Geometry: final body of the model. Coordinates: model frame, mm. A direction names the side the tool comes from. Give positions to 0.01 mm unless a question says otherwise; leave off trailing zeros. Loops run counter-clockwise (first coordinate to the right, second up) from the corner with the lowest first, then second, coordinate; pieces in that order, holes last.
```python
from build123d import *

# Parameters (mm, degrees)
BOSS_EXTRUDE1_DEPTH          = 29.21
SHELL1_T                     = -2.54
FILLET1_R                    = 6.35
BOSS_EXTRUDE2_DEPTH          = 38.1
SKETCH3_R                    = 2.8067
CUT_EXTRUDE1_DEPTH           = 4.7
CUT_EXTRUDE1_DRAFT           = -8
CUT_EXTRUDE1_PROFILE_2_DEPTH = 4.7
CUT_EXTRUDE1_PROFILE_2_DRAFT = -8
CUT_EXTRUDE1_PROFILE_3_DEPTH = 4.7
CUT_EXTRUDE1_PROFILE_3_DRAFT = -8
CUT_EXTRUDE1_PROFILE_4_DEPTH = 4.7
CUT_EXTRUDE1_PROFILE_4_DRAFT = -8
SKETCH5_W                    = 45.253999916
SKETCH5_H                    = 45.253999916
CUT_EXTRUDE5_DEPTH           = 38.1


with BuildPart() as part:
    # Sketch1 → Boss-Extrude1 (new, symmetric)
    with BuildSketch(Plane.XY):
        Polygon((-32.258, -32.258), (-32.258, -11.938), (-32.258, 11.938), (-32.258, 32.258), (32.258, 32.258), (32.258, -32.258), align=None)
    extrude(amount=BOSS_EXTRUDE1_DEPTH, both=True)

    # Shell1
    shell1_openings = [part.faces().sort_by_distance(p)[0] for p in [
        (0, 0, 29.21),
    ]]
    offset(amount=SHELL1_T, openings=shell1_openings, kind=Kind.INTERSECTION)

    # Fillet1
    fillet1_edges = [part.edges().sort_by_distance(p)[0] for p in [
        (-32.258, -32.258, 0),
        (-32.258, 32.258, 0),
        (32.258, 32.258, 0),
        (32.258, -32.258, 0),
        (-29.718, -29.718, 1.27),
        (29.718, -29.718, 1.27),
        (29.718, 29.718, 1.27),
        (-29.718, 29.718, 1.27),
        (-32.258, 0, -29.21),
        (0, 32.258, -29.21),
        (32.258, 0, -29.21),
        (0, -32.258, -29.21),
    ]]
    fillet(fillet1_edges, radius=FILLET1_R)

    # Sketch2 → Boss-Extrude2 (add)
    with BuildSketch(Plane.XY.offset(-26.67)):
        with BuildLine():
            Line((-20.828, -20.828), (-29.718, -20.828))
            Line((-29.718, -20.828), (-29.718, -23.368))
            ThreePointArc((-29.718, -23.368), (-27.858128061, -27.858128061), (-23.368, -29.718))
            Line((-23.368, -29.718), (-20.828, -29.718))
            Line((-20.828, -29.718), (-20.828, -20.828))
        make_face()
        with BuildLine():
            ThreePointArc((-29.718, 23.368), (-27.858128061, 27.858128061), (-23.368, 29.718))
            Line((-23.368, 29.718), (-20.828, 29.718))
            Line((-20.828, 29.718), (-20.828, 20.828))
            Line((-20.828, 20.828), (-29.718, 20.828))
            Line((-29.718, 20.828), (-29.718, 23.368))
        make_face()
        with BuildLine():
            ThreePointArc((29.718, 23.368), (27.858128061, 27.858128061), (23.368, 29.718))
            Line((23.368, 29.718), (20.828, 29.718))
            Line((20.828, 29.718), (20.828, 20.828))
            Line((20.828, 20.828), (29.718, 20.828))
            Line((29.718, 20.828), (29.718, 23.368))
        make_face()
        with BuildLine():
            ThreePointArc((23.368, -29.718), (27.858128061, -27.858128061), (29.718, -23.368))
            Line((29.718, -23.368), (29.718, -20.828))
            Line((29.718, -20.828), (20.828, -20.828))
            Line((20.828, -20.828), (20.828, -29.718))
            Line((20.828, -29.718), (23.368, -29.718))
        make_face()
    extrude(amount=BOSS_EXTRUDE2_DEPTH)


with BuildPart() as cut_extrude1_tool:
    # Sketch3 → Cut-Extrude1 (with draft: the straight prism first)
    with BuildSketch(Plane.XY.offset(11.43)):
        with Locations((-25.4, -25.4)):
            Circle(SKETCH3_R)
    extrude(amount=-CUT_EXTRUDE1_DEPTH)
    # Cut-Extrude1: the draft: its side faces are tilted about the plane it starts from
    cut_extrude1_sides = [cut_extrude1_tool.faces().sort_by_distance(p)[0] for p in [
        (-28.2067, -25.4, 9.08),
    ]]
    draft(cut_extrude1_sides, Plane.XY.offset(11.43), CUT_EXTRUDE1_DRAFT)


with BuildPart() as part_1:
    add(part.part)

    # Cut-Extrude1: cut by cut_extrude1_tool
    add(cut_extrude1_tool.part, mode=Mode.SUBTRACT)


with BuildPart() as cut_extrude1_profile_2_tool:
    # Sketch3 → Cut-Extrude1 profile 2 (with draft: the straight prism first)
    with BuildSketch(Plane.XY.offset(11.43)):
        with Locations((-25.4, 25.4)):
            Circle(SKETCH3_R)
    extrude(amount=-CUT_EXTRUDE1_PROFILE_2_DEPTH)
    # Cut-Extrude1 profile 2: the draft: its side faces are tilted about the plane it starts from
    cut_extrude1_profile_2_sides = [cut_extrude1_profile_2_tool.faces().sort_by_distance(p)[0] for p in [
        (-28.2067, 25.4, 9.08),
    ]]
    draft(cut_extrude1_profile_2_sides, Plane.XY.offset(11.43), CUT_EXTRUDE1_PROFILE_2_DRAFT)


with BuildPart() as part_2:
    add(part_1.part)

    # Cut-Extrude1 profile 2: cut by cut_extrude1_profile_2_tool
    add(cut_extrude1_profile_2_tool.part, mode=Mode.SUBTRACT)


with BuildPart() as cut_extrude1_profile_3_tool:
    # Sketch3 → Cut-Extrude1 profile 3 (with draft: the straight prism first)
    with BuildSketch(Plane.XY.offset(11.43)):
        with Locations((25.4, 25.4)):
            Circle(SKETCH3_R)
    extrude(amount=-CUT_EXTRUDE1_PROFILE_3_DEPTH)
    # Cut-Extrude1 profile 3: the draft: its side faces are tilted about the plane it starts from
    cut_extrude1_profile_3_sides = [cut_extrude1_profile_3_tool.faces().sort_by_distance(p)[0] for p in [
        (22.5933, 25.4, 9.08),
    ]]
    draft(cut_extrude1_profile_3_sides, Plane.XY.offset(11.43), CUT_EXTRUDE1_PROFILE_3_DRAFT)


with BuildPart() as part_3:
    add(part_2.part)

    # Cut-Extrude1 profile 3: cut by cut_extrude1_profile_3_tool
    add(cut_extrude1_profile_3_tool.part, mode=Mode.SUBTRACT)


with BuildPart() as cut_extrude1_profile_4_tool:
    # Sketch3 → Cut-Extrude1 profile 4 (with draft: the straight prism first)
    with BuildSketch(Plane.XY.offset(11.43)):
        with Locations((25.4, -25.4)):
            Circle(SKETCH3_R)
    extrude(amount=-CUT_EXTRUDE1_PROFILE_4_DEPTH)
    # Cut-Extrude1 profile 4: the draft: its side faces are tilted about the plane it starts from
    cut_extrude1_profile_4_sides = [cut_extrude1_profile_4_tool.faces().sort_by_distance(p)[0] for p in [
        (22.5933, -25.4, 9.08),
    ]]
    draft(cut_extrude1_profile_4_sides, Plane.XY.offset(11.43), CUT_EXTRUDE1_PROFILE_4_DRAFT)


with BuildPart() as part_4:
    add(part_3.part)

    # Cut-Extrude1 profile 4: cut by cut_extrude1_profile_4_tool
    add(cut_extrude1_profile_4_tool.part, mode=Mode.SUBTRACT)

    # Sketch5 → Cut-Extrude5 (cut)
    with BuildSketch(Plane.XY.offset(11.43)):
        Rectangle(SKETCH5_W, SKETCH5_H)
    extrude(amount=-CUT_EXTRUDE5_DEPTH, mode=Mode.SUBTRACT)


solid = part_4.part
```
Q1. Section query A-A, the plane x = -7.5. Return loops of the section in (y, z).
Q2. Mould query, pull axis Y, two halves, no side actions, for faces 1 (the face through (30.45, -0.36, -27.3)), 2 (the face through (-30.447, -30.348, 3.539)), 3 (the face through (-22.627, -22, -7)). Classes: +Y half, -Y half, draft (parallel to the pull), parting line (faces both ways), or undercut.
Q3. Section query B-B, the plane z = 1. Return loops of the section in (x, y).
Q4. Reachability of faces 4 (the face through (20.828, 26, -8)), 5 (the face through (3, -31, 29.21)) from +Z, -Z, +X, -X, +Y, -Y: full face, straight path, thin tool, end or side. Return the list, or none.
Q5. Pin query (flat end, axial travel): pin 1 Ø10 at (x, y) = (24, 8.5) entering from +Z; pin 2 Ø7 at (x, y) = (25, -27.5) entering from +Z; pin 3 Ø4.5 at (x, y) = (27, 23.5) entering from +Z. Return the tip coordinate at first contact, or that it passes through.
Q6. Material intervals for probe 1 along X at (y, z) = (11.5, -16); probe 2 along Y at (x, z) = (-25, 2), sorted ascending.
Resolved:
1. outline: (-32.26, -22.86) arc R6.35 ccw to (-25.91, -29.21) - (25.91, -29.21) arc R6.35 ccw to (32.26, -22.86) - (32.26, 29.21) - (29.72, 29.21) - (29.72, -26.67) - (-29.72, -26.67) - (-29.72, 29.21) - (-32.26, 29.21) - close
2. face 1: draft
2. face 2: -Y half
2. face 3: undercut
3. outline: (-32.26, -25.91) arc R6.35 ccw to (-25.91, -32.26) - (25.91, -32.26) arc R6.35 ccw to (32.26, -25.91) - (32.26, 25.91) arc R6.35 ccw to (25.91, 32.26) - (-25.91, 32.26) arc R6.35 ccw to (-32.26, 25.91) - close; hole (-29.72, -20.83) - (-22.63, -20.83) - (-22.63, -22.63) - (-20.83, -22.63) - (-20.83, -29.72) - (20.83, -29.72) - (20.83, -22.63) - (22.63, -22.63) - (22.63, -20.83) - (29.72, -20.83) - (29.72, 20.83) - (22.63, 20.83) - (22.63, 22.63) - (20.83, 22.63) - (20.83, 29.72) - (-20.83, 29.72) - (-20.83, 22.63) - (-22.63, 22.63) - (-22.63, 20.83) - (-29.72, 20.83) - close
4. face 4: +Z
4. face 5: +Z, +X, -X, +Y, -Y
5. pin 1: stops at z = -26.67
5. pin 2: stops at z = 29.21
5. pin 3: stops at z = 11.43
6. probe 1: x = -32.26 to -29.72, 29.72 to 32.26
6. probe 2: y = -32.26 to -20.83, 20.83 to 32.26
